from build123d import *

# Parameters (mm, degrees)
BOSS_EXTRUDE1_START = 142
SKETCH1_W           = 5
SKETCH1_H           = 16
BOSS_EXTRUDE1_DEPTH = 48
BOSS_EXTRUDE2_START = 148.9
SKETCH2_W           = 3.1
SKETCH2_H           = 4.1
BOSS_EXTRUDE2_DEPTH = 2.2
BOSS_EXTRUDE3_START = -1.75
BOSS_EXTRUDE3_DEPTH = 3.5
BOSS_EXTRUDE4_START = 59.4
SKETCH4_R           = 6.1
BOSS_EXTRUDE4_DEPTH = 1.7
BOSS_EXTRUDE5_START = 55.1
SKETCH5_R           = 3
BOSS_EXTRUDE5_DEPTH = 4.4
BOSS_EXTRUDE6_START = 59.4
SKETCH6_R           = 7.1
BOSS_EXTRUDE6_DEPTH = 1.7
BOSS_EXTRUDE7_START = 55.1
SKETCH7_R           = 3
BOSS_EXTRUDE7_DEPTH = 4.4


with BuildPart() as part:
    # Sketch1 → Boss-Extrude1 (new body)
    with BuildSketch(Plane.XY.offset(BOSS_EXTRUDE1_START)):
        with Locations((58.1, 0)):
            Rectangle(SKETCH1_W, SKETCH1_H)
    extrude(amount=BOSS_EXTRUDE1_DEPTH)


with BuildPart() as body_2:
    # Sketch2 → Boss-Extrude2 (new body)
    with BuildSketch(Plane.XY.offset(BOSS_EXTRUDE2_START)):
        with Locations((57.05, 0)):
            Rectangle(SKETCH2_W, SKETCH2_H)
    extrude(amount=BOSS_EXTRUDE2_DEPTH)


with BuildPart() as part_1:
    add(part.part)

    # Combine1: cut body 2
    add(body_2.part, mode=Mode.SUBTRACT)

    # Sketch3 → Boss-Extrude3 (add)
    with BuildSketch(Plane(origin=(0, 0, 0), x_dir=(1, 0, 0), z_dir=(0, 1, 0)).offset(BOSS_EXTRUDE3_START)):
        Polygon((58.8, -149.5), (58.8, -150.5), (52.8, -150.5), (52.8, -150.9), (52.2, -150.9), (51.4, -150.1), (51.4, -149.5), align=None)
    extrude(amount=BOSS_EXTRUDE3_DEPTH)


with BuildPart() as body_2_2:
    # Sketch4 → Boss-Extrude4 (new body)
    with BuildSketch(Plane(origin=(0, 0, 0), x_dir=(0, 0, -1), z_dir=(1, 0, 0)).offset(BOSS_EXTRUDE4_START)):
        with Locations((-165, 0)):
            Circle(SKETCH4_R)
    extrude(amount=BOSS_EXTRUDE4_DEPTH)


with BuildPart() as part_2:
    add(part_1.part)

    # Combine2: cut body 2 2
    add(body_2_2.part, mode=Mode.SUBTRACT)


with BuildPart() as body_2_3:
    # Sketch5 → Boss-Extrude5 (new body)
    with BuildSketch(Plane(origin=(0, 0, 0), x_dir=(0, 0, -1), z_dir=(1, 0, 0)).offset(BOSS_EXTRUDE5_START)):
        with Locations((-165, 0)):
            Circle(SKETCH5_R)
    extrude(amount=BOSS_EXTRUDE5_DEPTH)


with BuildPart() as part_3:
    add(part_2.part)

    # Combine3: cut body 2 3
    add(body_2_3.part, mode=Mode.SUBTRACT)


with BuildPart() as body_2_4:
    # Sketch6 → Boss-Extrude6 (new body)
    with BuildSketch(Plane(origin=(0, 0, 0), x_dir=(0, 0, -1), z_dir=(1, 0, 0)).offset(BOSS_EXTRUDE6_START)):
        with Locations((-181, 0)):
            Circle(SKETCH6_R)
    extrude(amount=BOSS_EXTRUDE6_DEPTH)


with BuildPart() as part_4:
    add(part_3.part)

    # Combine4: cut body 2 4
    add(body_2_4.part, mode=Mode.SUBTRACT)


with BuildPart() as body_2_5:
    # Sketch7 → Boss-Extrude7 (new body)
    with BuildSketch(Plane(origin=(0, 0, 0), x_dir=(0, 0, -1), z_dir=(1, 0, 0)).offset(BOSS_EXTRUDE7_START)):
        with Locations((-181, 0)):
            Circle(SKETCH7_R)
    extrude(amount=BOSS_EXTRUDE7_DEPTH)


with BuildPart() as part_5:
    add(part_4.part)

    # Combine5: cut body 2 5
    add(body_2_5.part, mode=Mode.SUBTRACT)


solid = part_5.part
Design review of the part built by this model. Coordinates are the model's own, in mm. A direction names the side the tool comes from. Give positions to 0.01 mm unless a question says otherwise; leave off trailing zeros. Order: outer loops, then holes, each group sorted by start corner. A loop starts at its lowest first (then second) coordinate and runs counter-clockwise, first axis right, second up. Notation, with made-up numbers: (-33, -16) - (-26, -16) arc R38 cw to (-26, 22) - close; hole circle Ø8 at (-27.5, 3.5). An arc over 180 degrees is marked (long way). Write item = value, one per line. Start each with the question number.
Q1. We need section C-C on y = 0. State how many separate pieces and enclosed holes the cut face has, plus the area to 3 significant figures.
Q2. Clearance check with flat-ended pins moving along their axes: pin 1 Ø1 at (x, y) = (55, 0.5) entering from -Z; pin 2 Ø3.5 at (y, z) = (0, 165) entering from +X; pin 3 Ø1 at (x, y) = (55, 0) entering from +Z. State where each tip first meets the part, or that it passes through.
Q3. To check wall thickness, follow L1, parallel to Z at x = 60.2, y = 0; L2, parallel to Z at x = 58.15, y = 0; L3, parallel to Y at x = 57.5, z = 181. State the ranges of each line that lie inside material, in increasing order. Write a range as from..to.
Q4. We need section D-D on z = 181. State the section outline as (x, y) points, plus the area to 3 significant figures.
Q5. We need section B-B on z = 165. State the section outline as (x, y) points, plus the area to 3 significant figures.
Q6. We need section A-A on x = 56.75. State the section outline as (y, z) points.
Q7. Mouldability with a two-part tool opening along Z and no side actions: class faces 4 (the face through (58, -8, 166)), 5 (the face through (58, 0, 190)), 6 (the face through (59.4, -3, 180)) as released by +Z, released by -Z, zero draft, split by the parting line, or undercut.
Q8. Tool access review of faces 1 (the face through (57.47, 0.9, 178.14)), 2 (the face through (55, 0, 149.5)), 3 (the face through (59.992, 0.268, 171.094)): name each direction out of +Z, -Z, +X, -X, +Y, -Y from which nothing blocks a thin tool from reaching the whole face with its end or side.
Working result:
q1.separate_pieces = 3
q1.enclosed_holes = 0
q1.area = 164 mm²
q2.pin_1 = 149.5
q2.pin_2 = through
q2.pin_3 = 150.5
q3.L1 = 142..158.9, 171.1..173.9, 188.1..190
q3.L2 = 142..148.9, 149.5..150.5, 151.1..162, 168..178, 184..190
q3.L3 = -8..-3, 3..8
q4.outline = (55.6, -8) - (60.6, -8) - (60.6, -7.1) - (59.4, -7.1) - (59.4, -3) - (55.6, -3) - close; (55.6, 3) - (59.4, 3) - (59.4, 7.1) - (60.6, 7.1) - (60.6, 8) - (55.6, 8) - close
q4.area = 40.2 mm²
q5.outline = (55.6, -8) - (60.6, -8) - (60.6, -6.1) - (59.4, -6.1) - (59.4, -3) - (55.6, -3) - close; (55.6, 3) - (59.4, 3) - (59.4, 6.1) - (60.6, 6.1) - (60.6, 8) - (55.6, 8) - close
q5.area = 42.6 mm²
q6.outline = (-8, 142) - (8, 142) - (8, 190) - (-8, 190) - close; (-1.75, 149.5) - (1.75, 149.5) - (1.75, 150.5) - (-1.75, 150.5) - close; hole circle Ø6 at (0, 165); hole circle Ø6 at (0, 181); hole (-2.05, 148.9) - (2.05, 148.9) - (2.05, 151.1) - (-2.05, 151.1) - close
q7.face_4 = zero draft
q7.face_5 = released by +Z
q7.face_6 = undercut
q8.face_1 = +X, -X
q8.face_2 = -X
q8.face_3 = +X
